Geometry: final body of the model. Coordinates: model frame, mm. A direction names the side the tool comes from. Give positions to 0.01 mm unless a question says otherwise; leave off trailing zeros. Write each loop counter-clockwise with the first axis right and the second up, starting at its lowest first coordinate (ties: lowest second). Pieces come first, ordered by that corner, then holes.
Autodesk Inventor part; units mm, degrees
ref_plane "YZ Plane" through (0, 0, 0) normal (1, 0, 0) x (0, 1, 0)
ref_plane "XZ Plane" through (0, 0, 0) normal (0, 1, 0) x (-1, 0, 0)
ref_plane "XY Plane" through (0, 0, 0) normal (0, 0, 1) x (1, 0, 0)
sketch "Skizze1" plane through (0, 0, 0) normal (0, 1, 0) x (-1, 0, 0)
  line L0 (8.9, -7.9) -> (-8.9, -7.9)
  line L1 (-8.9, -7.9) -> (-8.9, 7.9)
  line L2 (-8.9, 7.9) -> (8.9, 7.9)
  line L3 (8.9, 7.9) -> (8.9, -7.9)
  line L4 (12.46, 0) -> (-12.46, 0)
  line L5 (0, -11.06) -> (0, 11.06)
  line L6 (6, -5.1) -> (-6, -5.1)
  line L7 (-6, -5.1) -> (-6, 6.9)
  line L8 (-6, 6.9) -> (6, 6.9)
  line L9 (6, 6.9) -> (6, -5.1)
  circle A0 centre (7.65, -6.65) radius 0.75
  circle A1 centre (-7.65, -6.65) radius 0.75
  dimension "d0" = 17.8
  dimension "d1" = 15.8
  dimension "d3" = 12
  dimension "d4" = 12
  dimension "d5" = 1
  dimension "d15" = 1.5
  dimension "d16" = 1.25
  dimension "d17" = 1.25
extrude "Extrusion1" add sketch "Skizze1" along normal blind 1 contours L0 L5 L6 L9 L4 L3 | L0 L1 L4 L7 L6 L5 | L4 L9 L8 L5 L2 L3 | L6 L7 L4 L5 | L5 L4 L9 L6 | L4 L5 L8 L9 | L1 L2 L5 L8 L7 L4 | L4 L7 L8 L5 | A0 | A1
extrude "Extrusion2" add sketch "Skizze1" along normal blind 2 contours L6 L7 L4 L5 | L5 L4 L9 L6 | L4 L5 L8 L9 | L4 L7 L8 L5
sketch "Skizze2" plane through (0, 1, 0) normal (0, 1, 0) x (1, 0, 0)
  line L0 (-4.8872, 7.3) -> (-1.3872, 7.3)
  line L1 (-1.3872, 7.3) -> (-1.3872, 5.6)
  line L2 (-1.3872, 5.6) -> (-4.8872, 5.6)
  line L3 (-4.8872, 5.6) -> (-4.8872, 7.3)
  line L4 (6, 5.1) -> (-6, 5.1)
  point P0 (0, 0)
  dimension "d10" = 3.5
  dimension "d11" = 1.7
  dimension "d12" = 0.5
extrude "Extrusion3" add sketch "Skizze2" along normal blind 1.5
extrude "Extrusion4" cut sketch "Skizze1" along normal blind 1 contours A0 | A1
properties part number "GSMModul"
Q1. Pin query (flat end, axial travel): P1, Ø0.5, axis at x = 1, y = 1.5, coming from the +Z side; P2, Ø1, axis at x = 4, z = -2, coming from the +Y side; P3, Ø1.2, axis at x = -3.5, y = 1.5, coming from the +Z side; P4, Ø1.2, axis at x = -3.5, y = 2, coming from the -Z side. Return the tip coordinate at first contact, or that it passes through.
Filled sheet:
P1: stops at z = 6.9
P2: stops at y = 2
P3: stops at z = 7.9
P4: stops at z = -7.3
Q2. Pull-direction query (X, two-part tool) for faces 5 (the flat face through (-3, 2, -5.6)), 6 (the cylindrical face through (-8.34, 0.49, -6.36)), 7 (the cylindrical face through (7.813, 0.493, -5.918)), 8 (the flat face through (6, 1.5, 0.8)); classes: released by +X, released by -X, zero draft, split by the parting line, or undercut.
Filled sheet:
face 5: zero draft
face 6: undercut
face 7: undercut
face 8: released by +X
Q3. Section C-C on x = 7.65. Output: boundary loops of the cut face in (y, z).
Filled sheet:
outline: (0, -7.9) - (1, -7.9) - (1, -7.4) - (0, -7.4) - close; (0, -5.9) - (1, -5.9) - (1, 7.9) - (0, 7.9) - close
Q4. Ray query, line 1 along Z through (x, y) = (-7.65, 0.65); line 2 along X through (y, z) = (1.85, -1.5); line 3 along Y through (x, z) = (2, 1.5). Return the intervals inside material, ascending.
Filled sheet:
line 1: z = -7.9 to -7.4, -5.9 to 7.9
line 2: x = -6 to 6
line 3: y = 0 to 2
Q5. Section B-B on y = 1.7. Output: boundary loops of the cut face in (x, z).
Filled sheet:
outline: (-6, -5.1) - (6, -5.1) - (6, 6.9) - (-6, 6.9) - close; (-4.89, -7.3) - (-1.39, -7.3) - (-1.39, -5.6) - (-4.89, -5.6) - close
Q6. Section D-D on z = -2.5. Output: boundary loops of the cut face in (x, y).
Filled sheet:
outline: (-8.9, 0) - (8.9, 0) - (8.9, 1) - (6, 1) - (6, 2) - (-6, 2) - (-6, 1) - (-8.9, 1) - close
Q7. Section A-A on z = -6.65. Output: boundary loops of the cut face in (x, y), plus the area to 4 significant figures.
Filled sheet:
outline: (-8.9, 0) - (-8.4, 0) - (-8.4, 1) - (-8.9, 1) - close; (-6.9, 0) - (6.9, 0) - (6.9, 1) - (-1.39, 1) - (-1.39, 2.5) - (-4.89, 2.5) - (-4.89, 1) - (-6.9, 1) - close; (8.4, 0) - (8.9, 0) - (8.9, 1) - (8.4, 1) - close
area: 20.05 mm2
Q8. Access query for faces 1 (the flat face through (-4.887, 2, -6)), 2 (the flat face through (-6, 1.5, 1)), 3 (the flat face through (0, 2, 1)), 4 (the flat face through (-1.387, 2, -6)). Directions: +Z, -Z, +X, -X, +Y, -Y. A direction counts if a zero-diameter tool reaches every point of the face in a straight line with its end or side. Return the directions, or none.
Filled sheet:
face 1: -Z, -X, +Y
face 2: +Z, -Z, -X, +Y
face 3: +Z, +X, -X, +Y
face 4: -Z, +X, +Y
